Verification items for the finished model (mm, model axes). Round coordinates to 2 decimals unless told otherwise and drop trailing zeros. Write each loop counter-clockwise with the first axis right and the second up, starting at its lowest first coordinate (ties: lowest second). Pieces come first, ordered by that corner, then holes.
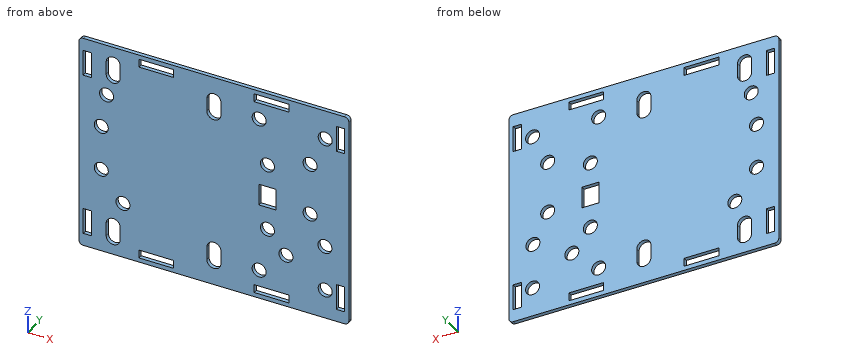
from build123d import *

# Parameters (mm, degrees)
SKETCH1_W                = 152.4
SKETCH1_H                = 127
BOSS_EXTRUDE1_DEPTH      = 2.3622
SKETCH9_R                = 4.15
CUT_EXTRUDE8_DEPTH       = 100.218294628
SKETCH16_R               = 4.15
CUT_EXTRUDE14_DEPTH      = 100.218294628
SKETCH26_W               = 10.16
SKETCH26_H               = 12.7
CUT_EXTRUDE26_DEPTH      = 100.218294628
SKETCH27_R               = 4.15
CUT_EXTRUDE27_DEPTH      = 100.218294628
SKETCH29_R               = 4.15
CUT_EXTRUDE28_DEPTH      = 100.218294628
SKETCH30_R               = 4.15
CUT_EXTRUDE29_DEPTH      = 100.218294628
SKETCH31_R               = 4.15
CUT_EXTRUDE30_DEPTH      = 100.218294628
SKETCH34_W               = 127
SKETCH34_H               = 2.3622
BOSS_EXTRUDE2_DEPTH      = 7.62
SKETCH38_W               = 88.9
SKETCH38_H               = 4.826
CUT_EXTRUDE34_DEPTH      = 7.62
SKETCH39_W               = 4.826
SKETCH39_H               = 15.24
CUT_EXTRUDE35_DEPTH      = 7.62
MIRROR15_COPY_1_SKETCH_W = 4.826
MIRROR15_COPY_1_SKETCH_H = 15.24
MIRROR15_COPY_1_DEPTH    = 7.62
CUT_EXTRUDE12_DEPTH      = 106.183755347
SKETCH40_W               = 47.752
SKETCH40_H               = 2.3622
BOSS_EXTRUDE3_DEPTH      = 4.826
FILLET2_R                = 2.54


with BuildPart() as part:
    # Sketch1 → Boss-Extrude1 (new body)
    with BuildSketch(Plane(origin=(0, 0, 0), x_dir=(1, 0, 0), z_dir=(0, 1, 0))):
        Rectangle(SKETCH1_W, SKETCH1_H)
    extrude(amount=BOSS_EXTRUDE1_DEPTH)

    # Sketch9 → Cut-Extrude8 (cut, through all)
    with BuildSketch(Plane.XZ):
        with Locations(Location((60.8584, 27.94, 0), (0, 0, 270))):
            Circle(SKETCH9_R)
        with Locations(Location((60.8584, -2.54, 0), (0, 0, 270))):
            Circle(SKETCH9_R)
    extrude(amount=-CUT_EXTRUDE8_DEPTH, mode=Mode.SUBTRACT)

    # Sketch16 → Cut-Extrude14 (cut, through all)
    with BuildSketch(Plane(origin=(0, 0, 0), x_dir=(-1, 0, 0), z_dir=(0, -1, 0))):
        with Locations(Location((-69.599893995, 19.704320306, 0), (0, 0, 90))):
            Circle(SKETCH16_R)
        with Locations(Location((-46.522565834, 32.264238523, 0), (0, 0, 90))):
            Circle(SKETCH16_R)
    extrude(amount=-CUT_EXTRUDE14_DEPTH, mode=Mode.SUBTRACT)

    # Sketch26 → Cut-Extrude26 (cut, through all)
    with BuildSketch(Plane(origin=(0, 2.3622, 0), x_dir=(1, 0, 0), z_dir=(0, 1, 0))):
        with Locations((35.56, 0)):
            Rectangle(SKETCH26_W, SKETCH26_H)
    extrude(amount=-CUT_EXTRUDE26_DEPTH, mode=Mode.SUBTRACT)

    # Sketch27 → Cut-Extrude27 (cut, through all)
    with BuildSketch(Plane.XZ):
        with Locations(Location((-59.831398438, 33.060447312, 0), (0, 0, 270))):
            Circle(SKETCH27_R)
        with Locations(Location((-50.09170874, -30.48, 0), (0, 0, 270))):
            Circle(SKETCH27_R)
    extrude(amount=-CUT_EXTRUDE27_DEPTH, mode=Mode.SUBTRACT)

    # Sketch29 → Cut-Extrude28 (cut, through all)
    with BuildSketch(Plane(origin=(0, 2.3622, 0), x_dir=(1, 0, 0), z_dir=(0, 1, 0))):
        with Locations(Location((35.56, 19.681240592, 0), (0, 0, 270))):
            Circle(SKETCH29_R)
        with Locations(Location((35.56, -19.681240592, 0), (0, 0, 270))):
            Circle(SKETCH29_R)
    extrude(amount=-CUT_EXTRUDE28_DEPTH, mode=Mode.SUBTRACT)

    # Sketch30 → Cut-Extrude29 (cut, through all)
    with BuildSketch(Plane(origin=(0, 2.3622, 0), x_dir=(1, 0, 0), z_dir=(0, 1, 0))):
        with Locations(Location((69.803274088, -46.355, 0), (0, 0, 270))):
            Circle(SKETCH30_R)
        with Locations(Location((30.63517528, -46.355, 0), (0, 0, 270))):
            Circle(SKETCH30_R)
    cut_extrude29 = extrude(amount=-CUT_EXTRUDE29_DEPTH, mode=Mode.SUBTRACT)

    # Mirror8: Cut-Extrude29 across plane
    add(cut_extrude29.mirror(Plane.XY), mode=Mode.SUBTRACT)

    # Sketch31 → Cut-Extrude30 (cut, through all)
    with BuildSketch(Plane(origin=(0, 2.3622, 0), x_dir=(1, 0, 0), z_dir=(0, 1, 0))):
        with Locations(Location((-62.942335235, -12.79551579, 0), (0, 0, 270))):
            Circle(SKETCH31_R)
        with Locations(Location((-62.942335235, 13.549600091, 0), (0, 0, 270))):
            Circle(SKETCH31_R)
    extrude(amount=-CUT_EXTRUDE30_DEPTH, mode=Mode.SUBTRACT)

    # Sketch34 → Boss-Extrude2 (add)
    with BuildSketch(Plane(origin=(76.2, 0, 0), x_dir=(0, 0, -1), z_dir=(1, 0, 0))):
        with Locations((0, 1.1811)):
            Rectangle(SKETCH34_W, SKETCH34_H)
    extrude(amount=BOSS_EXTRUDE2_DEPTH)

    # Sketch38 → Cut-Extrude34 (cut)
    with BuildSketch(Plane(origin=(0, 2.3622, 0), x_dir=(1, 0, 0), z_dir=(0, 1, 0))):
        with Locations((3.81, -58.547)):
            Rectangle(SKETCH38_W, SKETCH38_H)
    cut_extrude34 = extrude(amount=-CUT_EXTRUDE34_DEPTH, mode=Mode.SUBTRACT)

    # Mirror13: Cut-Extrude34 across plane
    add(cut_extrude34.mirror(Plane.XY), mode=Mode.SUBTRACT)

    # Sketch39 → Cut-Extrude35 (cut)
    with BuildSketch(Plane(origin=(0, 2.3622, 0), x_dir=(1, 0, 0), z_dir=(0, 1, 0))):
        with Locations((78.867, -48.514)):
            Rectangle(SKETCH39_W, SKETCH39_H)
    cut_extrude35 = extrude(amount=-CUT_EXTRUDE35_DEPTH, mode=Mode.SUBTRACT)

    # Mirror14: Cut-Extrude35 across plane
    add(cut_extrude35.mirror(Plane.XY), mode=Mode.SUBTRACT)

    # Mirror15: Cut-Extrude35 across plane
    add(cut_extrude35.mirror(Plane(origin=(3.81, 0, 0), x_dir=(0, 0, 1), z_dir=(1, 0, 0))), mode=Mode.SUBTRACT)

    # Mirror15 copy 1 sketch → Mirror15 copy 1 (cut)
    with BuildSketch(Plane(origin=(7.62, 2.3622, 0), x_dir=(-1, 0, 0), z_dir=(0, 1, 0))):
        with Locations((78.867, -48.514)):
            Rectangle(MIRROR15_COPY_1_SKETCH_W, MIRROR15_COPY_1_SKETCH_H)
    extrude(amount=-MIRROR15_COPY_1_DEPTH, mode=Mode.SUBTRACT)

    # Sketch13 → Cut-Extrude12 (cut, through all)
    with BuildSketch(Plane(origin=(0, 0, 0), x_dir=(-1, 0, 0), z_dir=(0, -1, 0))):
        with BuildLine():
            Line((60.052874771, -45.72), (60.052874771, -53.34))
            ThreePointArc((60.052874771, -53.34), (55.88, -57.512874771), (51.707125229, -53.34))
            Line((51.707125229, -53.34), (51.707125229, -45.72))
            ThreePointArc((51.707125229, -45.72), (55.88, -41.547125229), (60.052874771, -45.72))
        make_face()
        with BuildLine():
            Line((0.381, 49.403), (0.381, 41.783))
            ThreePointArc((0.381, 41.783), (-3.81, 37.592), (-8.001, 41.783))
            Line((-8.001, 41.783), (-8.001, 49.403))
            ThreePointArc((-8.001, 49.403), (-3.81, 53.594), (0.381, 49.403))
        make_face()
    cut_extrude12 = extrude(amount=-CUT_EXTRUDE12_DEPTH, mode=Mode.SUBTRACT)

    # Mirror16: Cut-Extrude12 across plane
    add(cut_extrude12.mirror(Plane.XY), mode=Mode.SUBTRACT)

    # Sketch40 → Boss-Extrude3 (add)
    with BuildSketch(Plane(origin=(0, 0, 60.96), x_dir=(-1, 0, 0), z_dir=(0, 0, -1))):
        with Locations((-3.81, 1.1811)):
            Rectangle(SKETCH40_W, SKETCH40_H)
    boss_extrude3 = extrude(amount=BOSS_EXTRUDE3_DEPTH)

    # Mirror17: Boss-Extrude3 across plane
    add(boss_extrude3.mirror(Plane.XY))

    # Fillet2
    fillet2_edges = [part.edges().sort_by_distance(p)[0] for p in [
        (83.82, 1.1811, -63.5),
        (-76.2, 1.1811, 63.5),
        (-76.2, 1.1811, -63.5),
        (83.82, 1.1811, 63.5),
    ]]
    fillet(fillet2_edges, radius=FILLET2_R)


solid = part.part
Q1. Sectioned sample at C-C (z = -21). Enter the section's corners in (x, y), plus the area to 3 significant figures.
Recorded:
outline: (-76.2, 0) - (31.63, 0) - (31.63, 2.36) - (-76.2, 2.36) - close; (39.49, 0) - (65.66, 0) - (65.66, 2.36) - (39.49, 2.36) - close; (73.54, 0) - (83.82, 0) - (83.82, 2.36) - (73.54, 2.36) - close
area: 341 mm2
Q2. Sectioned sample at D-D (y = 0.8). Give the number of separate pieces and of enclosed holes in the cut face, plus the area to 3 significant figures.
Recorded:
separate pieces: 1
enclosed holes: 27
area: 18,300 mm2
Q3. Sectioned sample at A-A (x = 3.81). Enter the section's corners in (y, z), plus the area to 3 significant figures.
Recorded:
outline: (0, -63.5) - (2.36, -63.5) - (2.36, -53.59) - (0, -53.59) - close; (0, -37.59) - (2.36, -37.59) - (2.36, 37.59) - (0, 37.59) - close; (0, 53.59) - (2.36, 53.59) - (2.36, 63.5) - (0, 63.5) - close
area: 224 mm2
Q4. Material ranges on line 1 along X through (y, z) = (0.85, 58); line 2 along Z through (x, y) = (41, 1.15); line 3 along X through (y, z) = (0.75, 27.94), recorded low to high.
Recorded:
line 1: x = -76.2 to -40.64, -20.07 to 27.69, 48.26 to 83.82
line 2: z = -63.5 to -60.96, -56.13 to 56.13, 60.96 to 63.5
line 3: x = -76.2 to 56.71, 65.01 to 83.82
Q5. Sectioned sample at B-B (x = 72). Enter the section's corners in (y, z), plus the area to 3 significant figures.
Recorded:
outline: (0, -63.5) - (2.36, -63.5) - (2.36, -49.88) - (0, -49.88) - close; (0, -42.83) - (2.36, -42.83) - (2.36, -23.09) - (0, -23.09) - close; (0, -16.32) - (2.36, -16.32) - (2.36, 42.83) - (0, 42.83) - close; (0, 49.88) - (2.36, 49.88) - (2.36, 63.5) - (0, 63.5) - close
area: 251 mm2
Q6. Depth check by flat-ended pin: P1, Ø6.5, axis at x = -50.09, z = -30.48, coming from the -Y side. Enter the tip coordinate at first touch or a pass-through.
Recorded:
P1: passes through
